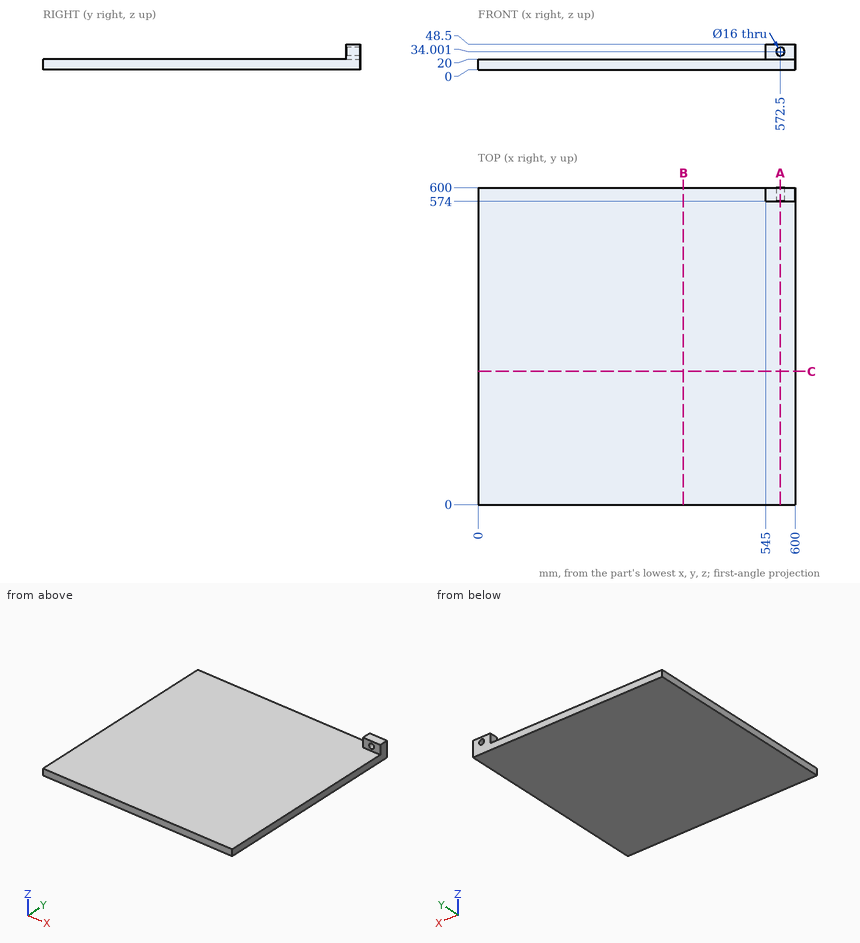
Here's the drawing with two shaded views (mm, measured from the low corner). I have some questions. Coordinates: 2 decimals unless noted, no trailing zeros. Order: outer loops, then holes, each group sorted by start corner. A loop starts at its lowest first (then second) coordinate and runs counter-clockwise, first axis right, second up. Notation, with made-up numbers: (44, -32) -> (80, -32) arc R12 cw to (80, -28) -> close; hole circle Ø11 at (33, 72). An arc over 180 degrees is marked (long way). One line per question, with ' | ' between items.
Q1. Imagine slicing it at A-A on x = 572.5. Please give me the cut outline in (y, z), and give its area (3 significant figures).
Return value:
outline: (0, 0) -> (600, 0) -> (600, 26) -> (574, 26) -> (574, 20) -> (0, 20) -> close; (574, 42) -> (600, 42) -> (600, 48.5) -> (574, 48.5) -> close | area: 12,300 mm²
Q2. Imagine slicing it at B-B on x = 388.5. Please give me the cut outline in (y, z).
Return value:
outline: (0, 0) -> (600, 0) -> (600, 20) -> (0, 20) -> close
Q3. I'm going to push flat-ended pins straight in: P1, Ø14, axis at x = 580, z = 28, coming from the -Y side; P2, Ø8, axis at x = 250, y = 220, coming from the +Z side; P3, Ø9.5, axis at x = 572.5, z = 34, coming from the +Y side; P4, Ø21, axis at y = 589.5, z = 40, coming from the -X side. Where does each tip first touch, or does it pass through?
Return value:
P1: y = 574 | P2: z = 20 | P3: through | P4: x = 545
Q4. If I drill on L1, parallel to Z at x = 572.5, y = 591.75; L2, parallel to Z at x = 538.5, y = 133, over which ranges is the centre line in solid material (lowest first)?
Return value:
L1: 0 to 26, 42 to 48.5 | L2: 0 to 20
